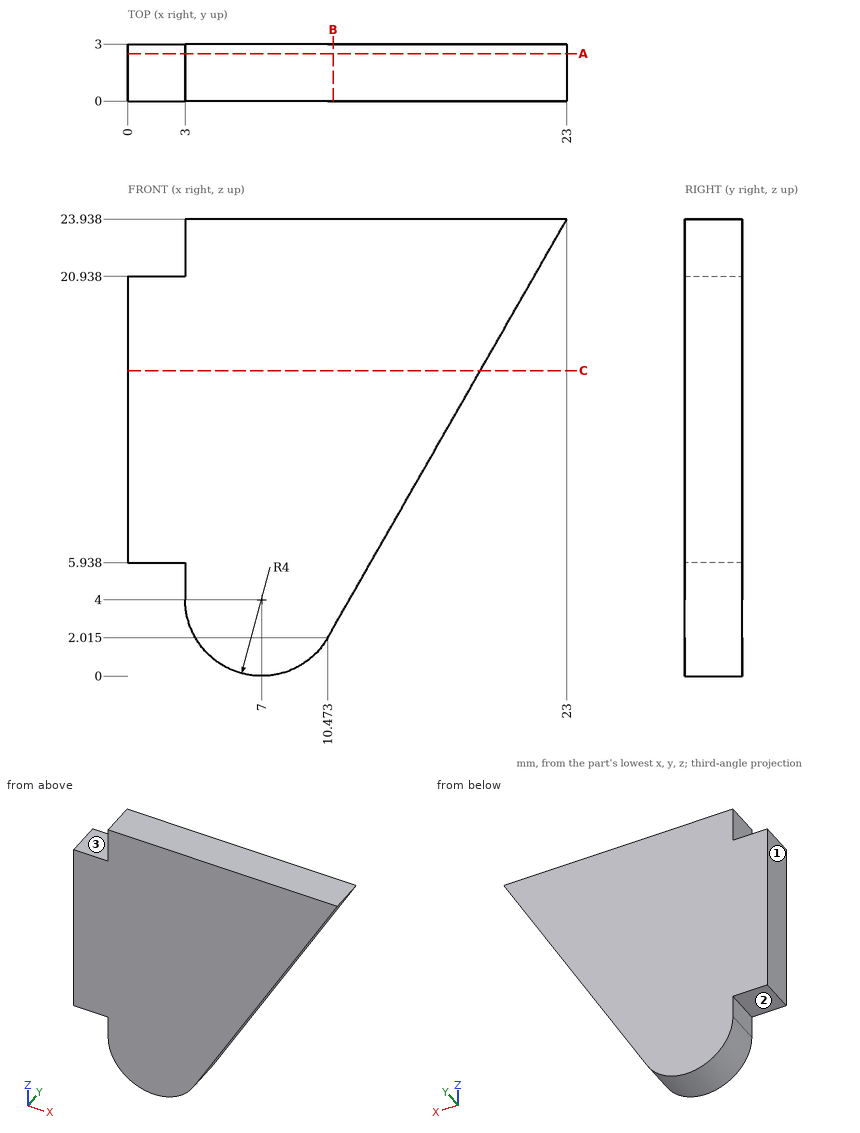
Answer from the drawing. Dimensions are ordinates in mm from the lowest x, y and z of the part. A direction names the side the tool comes from. Round coordinates to 2 decimals unless told otherwise and drop trailing zeros. Write each loop counter-clockwise with the first axis right and the second up, starting at its lowest first coordinate (ties: lowest second). Pieces come first, ordered by that corner, then holes. Notation, with made-up numbers: M 0,-3.5 L 59,-3.5 A5 cw 59,5.5 Z; hole C -27.5,61.5 d1. An arc over 180 degrees is marked long. Write each question's results on one line, items separated by ' | '. Start each with the question number.
Item 1: Which of the six approach directions +Z, -Z, +X, -X, +Y, -Y give full straight-line access (tool end or side, diameter ignored) to the marked faces 1, 2 and 3?
Item 2: Find section B-B on x = 10.75. Write down the section's boundary in (y, z).
Item 3: Straight lines are drawn through the part: probe 1 along Z at (x, y) = (2, 2.6); probe 2 along X at (y, z) = (1.5, 19.5) (1 decimal); probe 3 along Z at (x, y) = (18.5, 0.6) (1 decimal). For each, find the intervals that lie inside material, in ascending order.
Item 4: Find section A-A on y = 2.5. Write down the section's boundary in (x, z) (1 decimal), and give its area (3 significant figures).
Item 5: Find section C-C on z = 16. Write down the section's boundary in (x, y) (1 decimal).
Item 6: Given pin 1 Ø0.9 at (y, z) = (2, 22.5) entering from -X; pin 2 Ø1.5 at (x, y) = (1.5, 1) entering from +Z; pin 3 Ø1.5 at (x, y) = (15.5, 1.5) entering from -Z, each flat-ended and moving along its own axis, determine where each tip first touches the part or whether it passes through.
Answer block:
1) face 1: +Z, -Z, -X, +Y, -Y | face 2: -Z, -X, +Y, -Y | face 3: +Z, -X, +Y, -Y
2) outline: M 0,2.5 L 3,2.5 L 3,23.94 L 0,23.94 Z
3) probe 1: z = 5.94 to 20.94 | probe 2: x = 0 to 20.5 | probe 3: z = 16.1 to 23.9
4) outline: M 0,5.9 L 3,5.9 L 3,4 A4 ccw 10.5,2 L 23,23.9 L 3,23.9 L 3,20.9 L 0,20.9 Z | area: 356 mm²
5) outline: M 0,0 L 18.5,0 L 18.5,3 L 0,3 Z
6) pin 1: stops at x = 3 | pin 2: stops at z = 20.94 | pin 3: stops at z = 9.5
